Check sheet for the modelled part. Datum: model origin and axes. Units: mm. A direction names the side the tool comes from. Round coordinates to 2 decimals unless told otherwise and drop trailing zeros. Loops run counter-clockwise (first coordinate to the right, second up) from the corner with the lowest first, then second, coordinate; pieces in that order, holes last. Notation, with made-up numbers: M 42,70.25 L 73,70.25 A12 ccw 73,93.25 Z; hole C 76.25,51 d4. An arc over 180 degrees is marked long. Write item = value, one per line. Start each with the question number.
(1) Set-up check for faces 1 (the face through (0, 1, 1)), 2 (the face through (0, 2, -0.5)), 3 (the face through (0, 0, -0.5)): record each of +Z, -Z, +X, -X, +Y, -Y from which the full face is reachable in a straight line by a thin tool's end or side.
(2) Cross-section at D-D on z = 0.5. Record the boundary of the cut face in (x, y), plus the area to 3 significant figures.
(3) Cross-section at C-C on y = 6.5. Record the boundary of the cut face in (x, z).
(4) Cross-section at A-A on z = 0. Record the boundary of the cut face in (x, y), plus the area to 3 significant figures.
(5) Go/stop test with flat-tipped pins: P1, Ø2, axis at x = -1.5, y = 4.5, coming from the +Z side; P2, Ø1.5, axis at x = 2.5, y = -2, coming from the -Z side; P3, Ø1, axis at x = 1, z = 0.5, coming from the -Y side. Record where each tip stops, or that it passes through.
(6) Cross-section at B-B on x = -2.5. Record the boundary of the cut face in (y, z), plus the area to 3 significant figures.
(7) Scan lines: L1, parallel to X at y = 7, z = 0; L2, parallel to Y at x = 1.25, z = -0.5. Record each from-to range of solid material in increasing order. Write a range as from..to.
from build123d import *

# Parameters (mm, degrees)
IZIM1_R                          = 0.25
Y_KSEKLIK_EKSTR_ZYON1_DEPTH      = 2
IZIM3_R                          = 0.25
Y_KSEKLIK_EKSTR_ZYON3_DEPTH      = 6
Y_KSEKLIK_EKSTR_ZYON3_DEPTH_BACK = 5


with BuildPart() as part:
    # Çizim1 → Yükseklik-Ekstrüzyon1 (new body)
    with BuildSketch(Plane(origin=(0, 0, 0), x_dir=(1, 0, 0), z_dir=(0, 1, 0))):
        with BuildLine():
            Line((-3.477652227, 0.822347773), (-3.322347773, 0.977652227))
            ThreePointArc((-3.322347773, 0.977652227), (-3.297594249, 0.994192003), (-3.268395476, 1))
            Line((-3.268395476, 1), (-1.401604524, 1))
            ThreePointArc((-1.401604524, 1), (-1.372405751, 0.994192003), (-1.347652227, 0.977652227))
            Line((-1.347652227, 0.977652227), (-1.223952297, 0.853952297))
            ThreePointArc((-1.223952297, 0.853952297), (-1.17, 0.831604524), (-1.116047703, 0.853952297))
            Line((-1.116047703, 0.853952297), (-0.992347773, 0.977652227))
            ThreePointArc((-0.992347773, 0.977652227), (-0.967594249, 0.994192003), (-0.938395476, 1))
            Line((-0.938395476, 1), (0.935062143, 1))
            ThreePointArc((0.935062143, 1), (0.964260916, 0.994192003), (0.98901444, 0.977652227))
            Line((0.98901444, 0.977652227), (1.11271437, 0.853952297))
            ThreePointArc((1.11271437, 0.853952297), (1.166666667, 0.831604524), (1.220618963, 0.853952297))
            Line((1.220618963, 0.853952297), (1.344318894, 0.977652227))
            ThreePointArc((1.344318894, 0.977652227), (1.369072418, 0.994192003), (1.39827119, 1))
            Line((1.39827119, 1), (3.268395476, 1))
            ThreePointArc((3.268395476, 1), (3.297594249, 0.994192003), (3.322347773, 0.977652227))
            Line((3.322347773, 0.977652227), (3.477652227, 0.822347773))
            ThreePointArc((3.477652227, 0.822347773), (3.494192003, 0.797594249), (3.5, 0.768395476))
            Line((3.5, 0.768395476), (3.5, -0.768395476))
            ThreePointArc((3.5, -0.768395476), (3.494192003, -0.797594249), (3.477652227, -0.822347773))
            Line((3.477652227, -0.822347773), (3.322347773, -0.977652227))
            ThreePointArc((3.322347773, -0.977652227), (3.297594249, -0.994192003), (3.268395476, -1))
            Line((3.268395476, -1), (1.39827119, -1))
            ThreePointArc((1.39827119, -1), (1.369072418, -0.994192003), (1.344318894, -0.977652227))
            Line((1.344318894, -0.977652227), (1.220618963, -0.853952297))
            ThreePointArc((1.220618963, -0.853952297), (1.166666667, -0.831604524), (1.11271437, -0.853952297))
            Line((1.11271437, -0.853952297), (0.98901444, -0.977652227))
            ThreePointArc((0.98901444, -0.977652227), (0.964260916, -0.994192003), (0.935062143, -1))
            Line((0.935062143, -1), (-0.938395476, -1))
            ThreePointArc((-0.938395476, -1), (-0.967594249, -0.994192003), (-0.992347773, -0.977652227))
            Line((-0.992347773, -0.977652227), (-1.116047703, -0.853952297))
            ThreePointArc((-1.116047703, -0.853952297), (-1.17, -0.831604524), (-1.223952297, -0.853952297))
            Line((-1.223952297, -0.853952297), (-1.347652227, -0.977652227))
            ThreePointArc((-1.347652227, -0.977652227), (-1.372405751, -0.994192003), (-1.401604524, -1))
            Line((-1.401604524, -1), (-3.268395476, -1))
            ThreePointArc((-3.268395476, -1), (-3.297594249, -0.994192003), (-3.322347773, -0.977652227))
            Line((-3.322347773, -0.977652227), (-3.477652227, -0.822347773))
            ThreePointArc((-3.477652227, -0.822347773), (-3.494192003, -0.797594249), (-3.5, -0.768395476))
            Line((-3.5, -0.768395476), (-3.5, 0.768395476))
            ThreePointArc((-3.5, 0.768395476), (-3.494192003, 0.797594249), (-3.477652227, 0.822347773))
        make_face()
        Circle(IZIM1_R, mode=Mode.SUBTRACT)
        with Locations((-2.5, 0)):
            Circle(IZIM1_R, mode=Mode.SUBTRACT)
        with Locations((2.5, 0)):
            Circle(IZIM1_R, mode=Mode.SUBTRACT)
    extrude(amount=Y_KSEKLIK_EKSTR_ZYON1_DEPTH)

    # Çizim3 → Yükseklik-Ekstrüzyon3 (add, two sides)
    with BuildSketch(Plane(origin=(0, 2, 0), x_dir=(1, 0, 0), z_dir=(0, 1, 0))) as y_kseklik_ekstr_zyon3_sk:
        with Locations((-2.5, 0)):
            Circle(IZIM3_R)
        Circle(IZIM3_R)
        with Locations((2.5, 0)):
            Circle(IZIM3_R)
    extrude(amount=Y_KSEKLIK_EKSTR_ZYON3_DEPTH)
    extrude(y_kseklik_ekstr_zyon3_sk.sketch, amount=-Y_KSEKLIK_EKSTR_ZYON3_DEPTH_BACK)


solid = part.part
Result:
q1.face_1 = +Z, +X, -X, +Y, -Y
q1.face_2 = +Y
q1.face_3 = -Y
q2.outline = M -3.5,0 L 3.5,0 L 3.5,2 L -3.5,2 Z
q2.area = 14.0 mm^2
q3.outline = C -2.5,0 d0.5; C 0,0 d0.5; C 2.5,0 d0.5
q4.outline = M -3.5,0 L -2.75,0 L -2.75,-3 L -2.25,-3 L -2.25,0 L -0.25,0 L -0.25,-3 L 0.25,-3 L 0.25,0 L 2.25,0 L 2.25,-3 L 2.75,-3 L 2.75,0 L 3.5,0 L 3.5,2 L 2.75,2 L 2.75,8 L 2.25,8 L 2.25,2 L 0.25,2 L 0.25,8 L -0.25,8 L -0.25,2 L -2.25,2 L -2.25,8 L -2.75,8 L -2.75,2 L -3.5,2 Z
q4.area = 27.5 mm^2
q5.P1 = 0.25
q5.P2 = -0.25
q5.P3 = 0
q6.outline = M -3,-0.25 L 0,-0.25 L 0,-1 L 2,-1 L 2,-0.25 L 8,-0.25 L 8,0.25 L 2,0.25 L 2,1 L 0,1 L 0,0.25 L -3,0.25 Z
q6.area = 8.50 mm^2
q7.L1 = -2.75..-2.25, -0.25..0.25, 2.25..2.75
q7.L2 = 0..2
